Check sheet for the modelled part. Datum: model origin and axes. Units: mm. A direction names the side the tool comes from. Coordinates: 2 decimals unless noted, no trailing zeros. Answer as CSV lines item,"result".
from build123d import *

# Parameters (mm, degrees)
F_2020_PROFILE_DEPTH = 100


with BuildPart() as part:
    # Sketch1 → 2020 Profile (new, symmetric)
    with BuildSketch(Plane.XY):
        with BuildLine():
            Line((-3.655, 0), (-3.655, 2.383919339))
            ThreePointArc((-3.655, 2.383919339), (-3.693669197, 2.578322522), (-3.803789755, 2.743129583))
            Line((-3.803789755, 2.743129583), (-6.906870417, 5.846210245))
            ThreePointArc((-6.906870417, 5.846210245), (-7.071677478, 5.956330803), (-7.266080661, 5.995))
            Line((-7.266080661, 5.995), (-7.992, 5.995))
            ThreePointArc((-7.992, 5.995), (-8.351210245, 5.846210245), (-8.5, 5.487))
            Line((-8.5, 5.487), (-8.5, 3.138))
            ThreePointArc((-8.5, 3.138), (-8.648789755, 2.778789755), (-9.008, 2.63))
            Line((-9.008, 2.63), (-9.492, 2.63))
            ThreePointArc((-9.492, 2.63), (-9.851210245, 2.778789755), (-10, 3.138))
            Line((-10, 3.138), (-10, 8.5))
            ThreePointArc((-10, 8.5), (-9.560660172, 9.560660172), (-8.5, 10))
            Line((-8.5, 10), (-3.138, 10))
            ThreePointArc((-3.138, 10), (-2.778789755, 9.851210245), (-2.63, 9.492))
            Line((-2.63, 9.492), (-2.63, 9.008))
            ThreePointArc((-2.63, 9.008), (-2.778789755, 8.648789755), (-3.138, 8.5))
            Line((-3.138, 8.5), (-5.487, 8.5))
            ThreePointArc((-5.487, 8.5), (-5.846210245, 8.351210245), (-5.995, 7.992))
            Line((-5.995, 7.992), (-5.995, 7.266080661))
            ThreePointArc((-5.995, 7.266080661), (-5.956330803, 7.071677478), (-5.846210245, 6.906870417))
            Line((-5.846210245, 6.906870417), (-2.743129583, 3.803789755))
            ThreePointArc((-2.743129583, 3.803789755), (-2.578322522, 3.693669197), (-2.383919339, 3.655))
            Line((-2.383919339, 3.655), (0, 3.655))
            Line((0, 3.655), (2.383919339, 3.655))
            ThreePointArc((2.383919339, 3.655), (2.578322522, 3.693669197), (2.743129583, 3.803789755))
            Line((2.743129583, 3.803789755), (5.846210245, 6.906870417))
            ThreePointArc((5.846210245, 6.906870417), (5.956330803, 7.071677478), (5.995, 7.266080661))
            Line((5.995, 7.266080661), (5.995, 7.992))
            ThreePointArc((5.995, 7.992), (5.846210245, 8.351210245), (5.487, 8.5))
            Line((5.487, 8.5), (3.138, 8.5))
            ThreePointArc((3.138, 8.5), (2.778789755, 8.648789755), (2.63, 9.008))
            Line((2.63, 9.008), (2.63, 9.492))
            ThreePointArc((2.63, 9.492), (2.778789755, 9.851210245), (3.138, 10))
            Line((3.138, 10), (8.5, 10))
            ThreePointArc((8.5, 10), (9.560660172, 9.560660172), (10, 8.5))
            Line((10, 8.5), (10, 3.138))
            ThreePointArc((10, 3.138), (9.851210245, 2.778789755), (9.492, 2.63))
            Line((9.492, 2.63), (9.008, 2.63))
            ThreePointArc((9.008, 2.63), (8.648789755, 2.778789755), (8.5, 3.138))
            Line((8.5, 3.138), (8.5, 5.487))
            ThreePointArc((8.5, 5.487), (8.351210245, 5.846210245), (7.992, 5.995))
            Line((7.992, 5.995), (7.266080661, 5.995))
            ThreePointArc((7.266080661, 5.995), (7.071677478, 5.956330803), (6.906870417, 5.846210245))
            Line((6.906870417, 5.846210245), (3.803789755, 2.743129583))
            ThreePointArc((3.803789755, 2.743129583), (3.693669197, 2.578322522), (3.655, 2.383919339))
            Line((3.655, 2.383919339), (3.655, 0))
            Line((3.655, 0), (3.655, -2.383919339))
            ThreePointArc((3.655, -2.383919339), (3.693669197, -2.578322522), (3.803789755, -2.743129583))
            Line((3.803789755, -2.743129583), (6.906870417, -5.846210245))
            ThreePointArc((6.906870417, -5.846210245), (7.071677478, -5.956330803), (7.266080661, -5.995))
            Line((7.266080661, -5.995), (7.992, -5.995))
            ThreePointArc((7.992, -5.995), (8.351210245, -5.846210245), (8.5, -5.487))
            Line((8.5, -5.487), (8.5, -3.138))
            ThreePointArc((8.5, -3.138), (8.648789755, -2.778789755), (9.008, -2.63))
            Line((9.008, -2.63), (9.492, -2.63))
            ThreePointArc((9.492, -2.63), (9.851210245, -2.778789755), (10, -3.138))
            Line((10, -3.138), (10, -8.5))
            ThreePointArc((10, -8.5), (9.560660172, -9.560660172), (8.5, -10))
            Line((8.5, -10), (3.138, -10))
            ThreePointArc((3.138, -10), (2.778789755, -9.851210245), (2.63, -9.492))
            Line((2.63, -9.492), (2.63, -9.008))
            ThreePointArc((2.63, -9.008), (2.778789755, -8.648789755), (3.138, -8.5))
            Line((3.138, -8.5), (5.487, -8.5))
            ThreePointArc((5.487, -8.5), (5.846210245, -8.351210245), (5.995, -7.992))
            Line((5.995, -7.992), (5.995, -7.266080661))
            ThreePointArc((5.995, -7.266080661), (5.956330803, -7.071677478), (5.846210245, -6.906870417))
            Line((5.846210245, -6.906870417), (2.743129583, -3.803789755))
            ThreePointArc((2.743129583, -3.803789755), (2.578322522, -3.693669197), (2.383919339, -3.655))
            Line((2.383919339, -3.655), (0, -3.655))
            Line((0, -3.655), (-2.383919339, -3.655))
            ThreePointArc((-2.383919339, -3.655), (-2.578322522, -3.693669197), (-2.743129583, -3.803789755))
            Line((-2.743129583, -3.803789755), (-5.846210245, -6.906870417))
            ThreePointArc((-5.846210245, -6.906870417), (-5.956330803, -7.071677478), (-5.995, -7.266080661))
            Line((-5.995, -7.266080661), (-5.995, -7.992))
            ThreePointArc((-5.995, -7.992), (-5.846210245, -8.351210245), (-5.487, -8.5))
            Line((-5.487, -8.5), (-3.138, -8.5))
            ThreePointArc((-3.138, -8.5), (-2.778789755, -8.648789755), (-2.63, -9.008))
            Line((-2.63, -9.008), (-2.63, -9.492))
            ThreePointArc((-2.63, -9.492), (-2.778789755, -9.851210245), (-3.138, -10))
            Line((-3.138, -10), (-8.5, -10))
            ThreePointArc((-8.5, -10), (-9.560660172, -9.560660172), (-10, -8.5))
            Line((-10, -8.5), (-10, -3.138))
            ThreePointArc((-10, -3.138), (-9.851210245, -2.778789755), (-9.492, -2.63))
            Line((-9.492, -2.63), (-9.008, -2.63))
            ThreePointArc((-9.008, -2.63), (-8.648789755, -2.778789755), (-8.5, -3.138))
            Line((-8.5, -3.138), (-8.5, -5.487))
            ThreePointArc((-8.5, -5.487), (-8.351210245, -5.846210245), (-7.992, -5.995))
            Line((-7.992, -5.995), (-7.266080661, -5.995))
            ThreePointArc((-7.266080661, -5.995), (-7.071677478, -5.956330803), (-6.906870417, -5.846210245))
            Line((-6.906870417, -5.846210245), (-3.803789755, -2.743129583))
            ThreePointArc((-3.803789755, -2.743129583), (-3.693669197, -2.578322522), (-3.655, -2.383919339))
            Line((-3.655, -2.383919339), (-3.655, 0))
        make_face()
        with BuildLine():
            Line((-2.028687234, 1.848687546), (-1.848687546, 2.028687234))
            ThreePointArc((-1.848687546, 2.028687234), (-1.412354366, 2.11078896), (-1.177278935, 1.734136762))
            ThreePointArc((-1.177278935, 1.734136762), (-0.615818702, 2.003492782), (0, 2.096))
            ThreePointArc((0, 2.096), (0.615818702, 2.003492782), (1.177278935, 1.734136762))
            ThreePointArc((1.177278935, 1.734136762), (1.412354366, 2.11078896), (1.848687546, 2.028687234))
            Line((1.848687546, 2.028687234), (2.028687234, 1.848687546))
            ThreePointArc((2.028687234, 1.848687546), (2.11078896, 1.412354366), (1.734136762, 1.177278935))
            ThreePointArc((1.734136762, 1.177278935), (2.003492782, 0.615818702), (2.096, 0))
            ThreePointArc((2.096, 0), (2.003492782, -0.615818702), (1.734136762, -1.177278935))
            ThreePointArc((1.734136762, -1.177278935), (2.11078896, -1.412354366), (2.028687234, -1.848687546))
            Line((2.028687234, -1.848687546), (1.848687546, -2.028687234))
            ThreePointArc((1.848687546, -2.028687234), (1.412354366, -2.11078896), (1.177278935, -1.734136762))
            ThreePointArc((1.177278935, -1.734136762), (0.615818702, -2.003492782), (0, -2.096))
            ThreePointArc((0, -2.096), (-0.615818702, -2.003492782), (-1.177278935, -1.734136762))
            ThreePointArc((-1.177278935, -1.734136762), (-1.412354366, -2.11078896), (-1.848687546, -2.028687234))
            Line((-1.848687546, -2.028687234), (-2.028687234, -1.848687546))
            ThreePointArc((-2.028687234, -1.848687546), (-2.11078896, -1.412354366), (-1.734136762, -1.177278935))
            ThreePointArc((-1.734136762, -1.177278935), (-2.003492782, -0.615818702), (-2.096, 0))
            ThreePointArc((-2.096, 0), (-2.003492782, 0.615818702), (-1.734136762, 1.177278935))
            ThreePointArc((-1.734136762, 1.177278935), (-2.11078896, 1.412354366), (-2.028687234, 1.848687546))
        make_face(mode=Mode.SUBTRACT)
    extrude(amount=F_2020_PROFILE_DEPTH, both=True)


solid = part.part
1) Depth check by flat-ended pin: P1, Ø1.4, axis at y = 1, z = 16, coming from the +X side (3 decimals); P2, Ø3, axis at x = 1.5, y = 6.5, coming from the -Z side; P3, Ø3, axis at x = 0, z = 59.5, coming from the +Y side (3 decimals). Enter the tip coordinate at first touch or a pass-through.
Answer key:
P1,"stops at x = 3.655"
P2,"passes through"
P3,"stops at y = 3.655"
2) Mould release check, pull along Y, two halves, no side actions. Record for faces 1 (the face through (5.38, 4.32, 1.4)), 2 (the face through (6, -10, 1)), 3 (the face through (-10, 6, 1)), 4 (the face through (6, 10, 1)): pulls with the +Y half, pulls with the -Y half, needs draft (parallel to the pull), parting line crosses it, or undercut.
Answer key:
face 1,"undercut"
face 2,"pulls with the -Y half"
face 3,"needs draft"
face 4,"pulls with the +Y half"
3) Tool access check on faces 5 (the face through (5.33, -4.27, 1.4)), 6 (the face through (0, -3.655, 1)), 7 (the face through (3.655, 0, 1)), 8 (the face through (-3.655, 0, 1)). Record the directions out of +Z, -Z, +X, -X, +Y, -Y that give a thin tool (end or side, any length) a straight path to the whole face; none if there is none.
Answer key:
face 5,"+Z, -Z"
face 6,"+Z, -Z, -Y"
face 7,"+Z, -Z, +X"
face 8,"+Z, -Z, -X"
4) Thickness scan on line 1 along Y through (x, z) = (-4.75, -82.5); line 2 along Y through (x, z) = (0.25, 53) (3 decimals); line 3 along X through (y, z) = (5.5, 82). Record the ranges inside material, lowest first.
Answer key:
line 1,"y = -10 to -8.5, -5.81 to -3.69, 3.69 to 5.81, 8.5 to 10"
line 2,"y = -3.655 to -2.081, 2.081 to 3.655"
line 3,"x = -10 to -8.5, -6.56 to -4.44, 4.44 to 6.56, 8.5 to 10"
